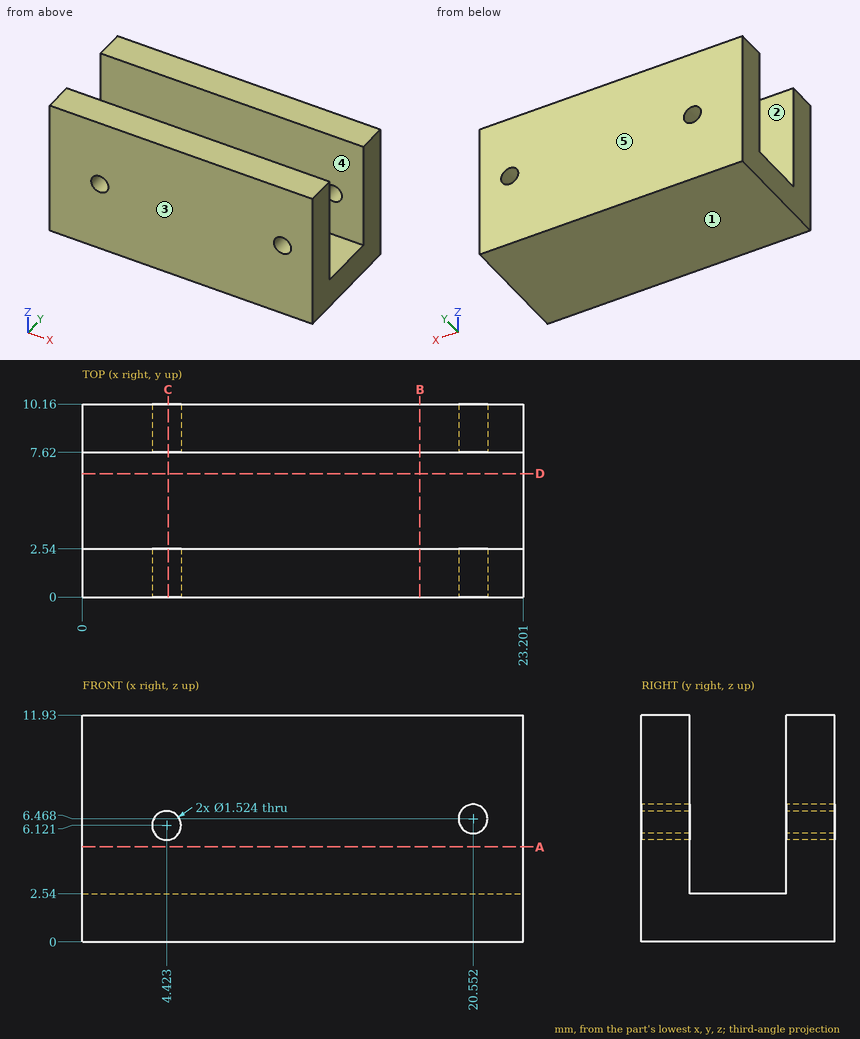
Part print with two shaded views. Sizes in mm from the minimum x, y, z corner. A direction names the side the tool comes from. Coordinates: 2 decimals unless noted, no trailing zeros. Write each loop counter-clockwise with the first axis right and the second up, starting at its lowest first coordinate (ties: lowest second). Pieces come first, ordered by that corner, then holes. Notation, with made-up numbers: (26, 7.5) - (66, 7.5) arc R15 ccw to (66, 11.5) - close; hole circle Ø5 at (-37, 59.25). An arc over 180 degrees is marked (long way). Put each result on its own line as item: value.
1. 3-axis set-ups, long thin cutter, end or side, ignore diameter. For the marked faces 1 and 2: which of +Z, -Z, +X, -X, +Y, -Y reach the whole face in a straight line?
Final values:
face 1: -Z, +X, -X, +Y, -Y
face 2: +Z, +X, -X
2. Probe line 1 along Y through (x, z) = (16.25, 6.25); line 2 along Z through (x, y) = (12, 6.5); line 3 along Z through (x, y) = (4.75, 1.5). List the from-to ranges inside material, lowest first. Write a range as [from, to].
Final values:
line 1: y = [0, 2.54], [7.62, 10.16]
line 2: z = [0, 2.54]
line 3: z = [0, 5.43], [6.81, 11.93]
3. Flat gauge pin, fed straight in: pin 1 Ø1.4 at (x, z) = (4.42, 6.12) entering from +Y. Where does the tip first touch, or does it go through?
Final values:
pin 1: passes through
4. Two-plate mould, pull along Y, no slides. Class the marked faces 3, 4 and 5: +Y half, -Y half, draft (parallel to the pull), parting line (faces both ways), or undercut.
Final values:
face 3: -Y half
face 4: undercut
face 5: +Y half
5. Band-saw the part on C-C (x = 4.5). Write the cut outline in (y, z), then the cut area to 3 significant figures.
Final values:
outline: (0, 0) - (10.16, 0) - (10.16, 5.36) - (7.62, 5.36) - (7.62, 2.54) - (2.54, 2.54) - (2.54, 5.36) - (0, 5.36) - close; (0, 6.88) - (2.54, 6.88) - (2.54, 11.93) - (0, 11.93) - close; (7.62, 6.88) - (10.16, 6.88) - (10.16, 11.93) - (7.62, 11.93) - close
area: 65.8 mm²
6. Band-saw the part on A-A (z = 5). Write the cut outline in (x, y), then the cut area to 3 significant figures.
Final values:
outline: (0, 0) - (23.2, 0) - (23.2, 2.54) - (0, 2.54) - close; (0, 7.62) - (23.2, 7.62) - (23.2, 10.16) - (0, 10.16) - close
area: 118 mm²
7. Band-saw the part on D-D (y = 6.5). Write the cut outline in (x, z).
Final values:
outline: (0, 0) - (23.2, 0) - (23.2, 2.54) - (0, 2.54) - close
8. Band-saw the part on B-B (x = 17.75). Write the cut outline in (y, z).
Final values:
outline: (0, 0) - (10.16, 0) - (10.16, 11.93) - (7.62, 11.93) - (7.62, 2.54) - (2.54, 2.54) - (2.54, 11.93) - (0, 11.93) - close
